Check sheet for the drawn part. Datum: minimum x, y, z corner. Units: mm. Coordinates: 2 decimals unless noted, no trailing zeros. Write each loop counter-clockwise with the first axis right and the second up, starting at its lowest first coordinate (ties: lowest second). Pieces come first, ordered by that corner, then holes. Notation, with made-up numbers: (32, -30.75) -> (45, -30.75) arc R30 ccw to (45, 2.25) -> close; hole circle Ø5 at (20.25, 2). An arc over 180 degrees is marked (long way). Answer in a Markdown table with one row per item. Add a question column.
1. Cross-section at C-C on z = 1.85. Record the cut outline in (x, y), and give its area (3 significant figures).
2. Cross-section at B-B on x = 21. Record the cut outline in (y, z), and give its area (3 significant figures).
3. Scan lines: L1, parallel to X at y = 42, z = 2.15; L2, parallel to Y at x = 105.5, z = 1.05; L3, parallel to Y at x = 69, z = 2.5. Record each from-to range of solid material in increasing order. Write a range as from..to.
4. Depth check by flat-ended pin: P1, Ø6, axis at x = 93.5, y = 39.5, coming from the -Z side (1 decimal). Enter the tip coordinate at first touch or a pass-through.
5. Cross-section at A-A on y = 35. Record the cut outline in (x, z), and give its area (3 significant figures).
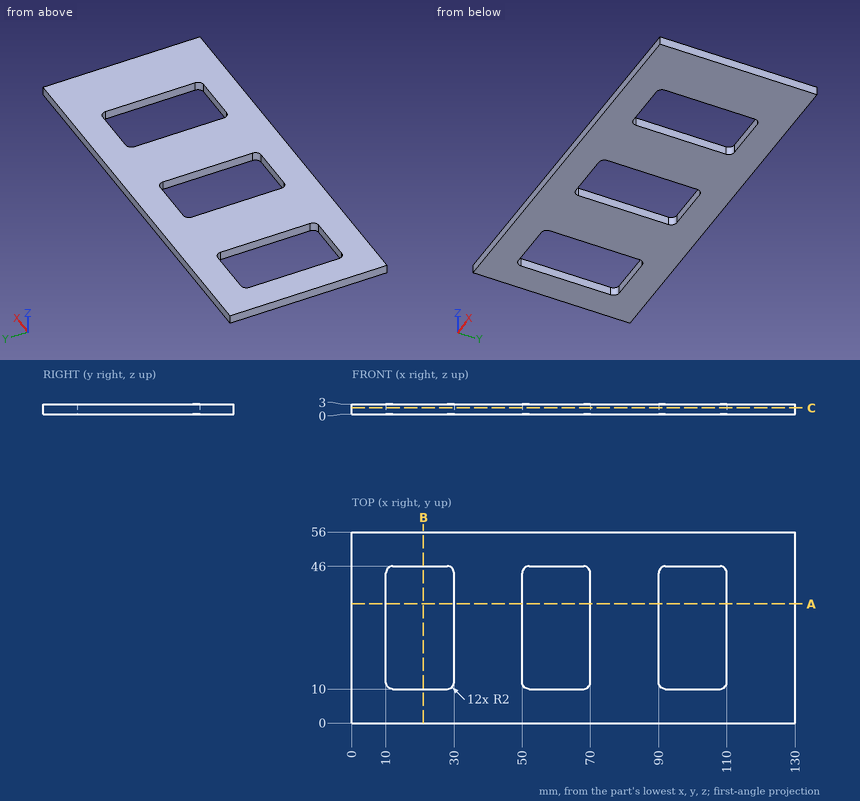
Results found:
| question | item | result |
|---|---|---|
| 1 | outline | (0, 0) -> (130, 0) -> (130, 56) -> (0, 56) -> close; hole (10, 12) arc R2 ccw to (12, 10) -> (28, 10) arc R2 ccw to (30, 12) -> (30, 44) arc R2 ccw to (28, 46) -> (12, 46) arc R2 ccw to (10, 44) -> close; hole (50, 12) arc R2 ccw to (52, 10) -> (68, 10) arc R2 ccw to (70, 12) -> (70, 44) arc R2 ccw to (68, 46) -> (52, 46) arc R2 ccw to (50, 44) -> close; hole (90, 12) arc R2 ccw to (92, 10) -> (108, 10) arc R2 ccw to (110, 12) -> (110, 44) arc R2 ccw to (108, 46) -> (92, 46) arc R2 ccw to (90, 44) -> close |
| 1 | area | 5,130 mm^2 |
| 2 | outline | (0, 0) -> (10, 0) -> (10, 3) -> (0, 3) -> close; (46, 0) -> (56, 0) -> (56, 3) -> (46, 3) -> close |
| 2 | area | 60.0 mm^2 |
| 3 | L1 | x = 0..10, 30..50, 70..90, 110..130 |
| 3 | L2 | y = 0..10, 46..56 |
| 3 | L3 | y = 0..10.27, 45.73..56 |
| 4 | P1 | passes through |
| 5 | outline | (0, 0) -> (10, 0) -> (10, 3) -> (0, 3) -> close; (30, 0) -> (50, 0) -> (50, 3) -> (30, 3) -> close; (70, 0) -> (90, 0) -> (90, 3) -> (70, 3) -> close; (110, 0) -> (130, 0) -> (130, 3) -> (110, 3) -> close |
| 5 | area | 210 mm^2 |
